Part model, mm, in its own coordinate system. Coordinates: 2 decimals unless noted, no trailing zeros. Loops run counter-clockwise (first coordinate to the right, second up) from the corner with the lowest first, then second, coordinate; pieces in that order, holes last. Notation, with made-up numbers: M -29.75,-34.5 L -20.75,-34.5 A16 cw -20.75,-29.5 Z; hole C 6,78.25 d2. An arc over 180 degrees is marked long. Answer as a JSON object with one key per item and string values. Group by question number.
1. Saw through at B-B on y = 17.25. Write the cut outline in (x, z).
2. Drop a flat-ended pin along its axis: pin 1 Ø4 at (x, z) = (11.5, -2.5) entering from -Y. Give the stop position or say it passes through.
3. Saw through at A-A on x = 12.5. Write the cut outline in (y, z).
4. Drill centre lines: L1, parallel to Y at x = 3.5, z = -1.75; L2, parallel to Z at x = 13.5, y = 18.25. Where is each one in solid material? Low to high.
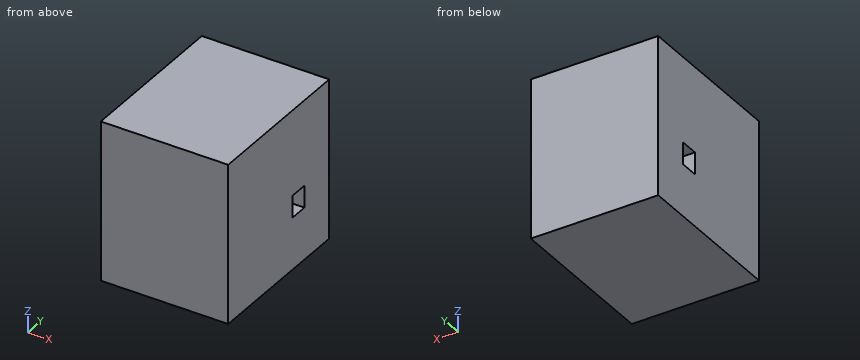
from build123d import *

# Parameters (mm, degrees)
F0_W     = 20
F0_H     = 25
F1_DEPTH = 12.5000001863
F3_W     = 2.9370598495
F3_H     = 3.4478511661
F4_DEPTH = 25


with BuildPart() as f1:
    # F0 (on Top) → F1 (new body, symmetric)
    with BuildSketch(Plane.XY):
        with Locations((10, 12.5)):
            Rectangle(F0_W, F0_H)
    extrude(amount=F1_DEPTH, both=True)

    # F3 (on face) → F4 (cut)
    with BuildSketch(Plane.YZ.offset(20)):
        with Locations((17.3844564706, -2.6178145781)):
            Rectangle(F3_W, F3_H)
    extrude(amount=-F4_DEPTH, mode=Mode.SUBTRACT)


solid = f1.part
Outcome:
{
 "1": {"outline": "M 0,-12.5 L 20,-12.5 L 20,-4.34 L 0,-4.34 Z; M 0,-0.89 L 20,-0.89 L 20,12.5 L 0,12.5 Z"},
 "2": {"pin 1": "stops at y = 0"},
 "3": {"outline": "M 0,-12.5 L 25,-12.5 L 25,12.5 L 0,12.5 Z; hole M 15.92,-4.34 L 18.85,-4.34 L 18.85,-0.89 L 15.92,-0.89 Z"},
 "4": {"L1": "y = 0 to 15.92, 18.85 to 25", "L2": "z = -12.5 to -4.34, -0.89 to 12.5"}
}
